```python
from build123d import *

# Parameters (mm, degrees)
BASE_EXTRUDE_DEPTH         = 31.1
SKETCH2_W                  = 13.52
SKETCH2_H                  = 6.37
BOSS_EXTRUDE1_DEPTH        = 8.41
SKETCH3_R                  = 1.545
BASE_MOUNTING_HOLE_1_DEPTH = 35.931591719
SKETCH5_R                  = 1.1305
FACE_MOUNTING_HOLES_DEPTH  = 37.029023023
SHELL_AROUND_PINS_DEPTH    = 5.7
SHELL1_START               = 0.44
SHELL1_DEPTH               = 18.2
SHELL1_START_2             = 8.5
SHELL1_2_OUTLINE_W         = 11.54
SHELL1_2_OUTLINE_H         = 30.22
SHELL1_2_OUTLINE_R         = 1.5705
SHELL1_2_DEPTH             = 4
SHELL1_START_3             = 12.5
SHELL1_3_DEPTH             = 6.14
SHELL1_START_4             = 5.3050001
SHELL1_4_DEPTH             = 3.1949999
SHELL1_5_DEPTH             = 0.8949999
SHELL1_START_5             = 0.09
SHELL1_6_OUTLINE_W         = 5.49
SHELL1_6_OUTLINE_H         = 12.64
SHELL1_6_DEPTH             = 0.35
SHELL1_7_DEPTH             = 2.29
BOSS_EXTRUDE2_DEPTH        = 3.9
BOSS_EXTRUDE3_DEPTH        = 6.24
SKETCH9_R                  = 0.675
CUT_EXTRUDE1_DEPTH         = 6.4


with BuildPart() as part:
    # Sketch1 → Base-Extrude (new body)
    with BuildSketch(Plane.XY):
        Polygon((0, 0), (12.94, 0), (12.94, 12.42), (8.06, 12.42), (8.06, 3.17), (0, 3.17), align=None)
    extrude(amount=BASE_EXTRUDE_DEPTH)

    # Sketch2 → Boss-Extrude1 (add)
    with BuildSketch(Plane.ZY.offset(-8.06)):
        with Locations((15.55, 6.355)):
            Rectangle(SKETCH2_W, SKETCH2_H)
    extrude(amount=BOSS_EXTRUDE1_DEPTH)

    # Sketch3 → Base Mounting Hole 1 (cut, through all)
    with BuildSketch(Plane(origin=(0, 3.17, 0), x_dir=(-1, 0, 0), z_dir=(0, 1, 0))):
        with Locations((-3.32, 3.05)):
            Circle(SKETCH3_R)
        with Locations((-3.32, 28.05)):
            Circle(SKETCH3_R)
    extrude(amount=-BASE_MOUNTING_HOLE_1_DEPTH, mode=Mode.SUBTRACT)

    # Sketch5 → Face Mounting Holes (cut, through all)
    with BuildSketch(Plane(origin=(12.94, 0, 0), x_dir=(0, 0, -1), z_dir=(1, 0, 0))):
        with Locations((-3.05, 6.04)):
            Circle(SKETCH5_R)
        with Locations((-28.05, 6.04)):
            Circle(SKETCH5_R)
    extrude(amount=-FACE_MOUNTING_HOLES_DEPTH, mode=Mode.SUBTRACT)

    # Sketch6 → Shell around Pins (add)
    with BuildSketch(Plane(origin=(12.94, 0, 0), x_dir=(0, 0, -1), z_dir=(1, 0, 0))):
        with BuildLine():
            Line((-22.906967712, 11.06), (-8.213032288, 11.06))
            ThreePointArc((-8.213032288, 11.06), (-7.106786662, 10.573025476), (-6.718825618, 9.428294154))
            Line((-6.718825618, 9.428294154), (-7.309392629, 2.728294154))
            ThreePointArc((-7.309392629, 2.728294154), (-7.790573821, 1.753754374), (-8.803599298, 1.36))
            Line((-8.803599298, 1.36), (-22.316400702, 1.36))
            ThreePointArc((-22.316400702, 1.36), (-23.329426179, 1.753754374), (-23.810607371, 2.728294154))
            Line((-23.810607371, 2.728294154), (-24.401174382, 9.428294154))
            ThreePointArc((-24.401174382, 9.428294154), (-24.013213338, 10.573025476), (-22.906967712, 11.06))
        make_face()
    extrude(amount=SHELL_AROUND_PINS_DEPTH)

    # Shell1: read off the stored shape, not the designer's step
    # Shell1 outline → Shell1 (cut)
    with BuildSketch(Plane.YZ.offset(SHELL1_START)):
        with BuildLine():
            Line((2.73, 21.87), (2.73, 23.368398801))
            ThreePointArc((2.73, 23.368398801), (2.06583377, 23.018469075), (1.8, 22.316400702))
            Line((1.8, 22.316400702), (1.8, 8.803599298))
            ThreePointArc((1.8, 8.803599298), (2.06583377, 8.101530925), (2.73, 7.751601199))
            Line((2.73, 7.751601199), (2.73, 9.23))
            Line((2.73, 9.23), (9.1, 9.23))
            Line((9.1, 9.23), (9.1, 21.87))
            Line((9.1, 21.87), (2.73, 21.87))
        make_face()
    extrude(amount=SHELL1_DEPTH, mode=Mode.SUBTRACT)

    # Shell1 2 outline → Shell1 2 (cut)
    with BuildSketch(Plane.YZ.offset(SHELL1_START_2)):
        with Locations((6.21, 15.55)):
            Rectangle(SHELL1_2_OUTLINE_W, SHELL1_2_OUTLINE_H)
        with Locations((6.04, 3.05)):
            Circle(SHELL1_2_OUTLINE_R, mode=Mode.SUBTRACT)
        with Locations((6.04, 28.05)):
            Circle(SHELL1_2_OUTLINE_R, mode=Mode.SUBTRACT)
        with BuildLine():
            ThreePointArc((1.8, 22.316400702), (2.06583377, 23.018469075), (2.73, 23.368398801))
            Line((2.73, 23.368398801), (2.73, 21.87))
            Line((2.73, 21.87), (9.1, 21.87))
            Line((9.1, 21.87), (9.1, 9.23))
            Line((9.1, 9.23), (2.73, 9.23))
            Line((2.73, 9.23), (2.73, 7.751601199))
            ThreePointArc((2.73, 7.751601199), (2.06583377, 8.101530925), (1.8, 8.803599298))
            Line((1.8, 8.803599298), (1.8, 22.316400702))
        make_face(mode=Mode.SUBTRACT)
    extrude(amount=SHELL1_2_DEPTH, mode=Mode.SUBTRACT)

    # Shell1 3 outline → Shell1 3 (cut)
    with BuildSketch(Plane.YZ.offset(SHELL1_START_3)):
        with BuildLine():
            ThreePointArc((2.766927869, 23.372306748), (2.74844682, 23.370514495), (2.73, 23.368398801))
            Line((2.73, 23.368398801), (2.73, 21.87))
            Line((2.73, 21.87), (9.1, 21.87))
            Line((9.1, 21.87), (9.1, 9.23))
            Line((9.1, 9.23), (2.73, 9.23))
            Line((2.73, 9.23), (2.73, 7.751601199))
            ThreePointArc((2.73, 7.751601199), (2.74844682, 7.749485505), (2.766927869, 7.747693252))
            Line((2.766927869, 7.747693252), (9.466927869, 7.157126241))
            ThreePointArc((9.466927869, 7.157126241), (10.275871337, 7.431285379), (10.62, 8.213032288))
            Line((10.62, 8.213032288), (10.62, 22.906967712))
            ThreePointArc((10.62, 22.906967712), (10.275871337, 23.688714621), (9.466927869, 23.962873759))
            Line((9.466927869, 23.962873759), (2.766927869, 23.372306748))
        make_face()
    extrude(amount=SHELL1_3_DEPTH, mode=Mode.SUBTRACT)

    # Shell1 4 outline → Shell1 4 (cut)
    with BuildSketch(Plane.YZ.offset(SHELL1_START_4)):
        with BuildLine():
            Line((2.73, 23.368398801), (2.73, 30.66))
            Line((2.73, 30.66), (0.44, 30.66))
            Line((0.44, 30.66), (0.44, 0.44))
            Line((0.44, 0.44), (2.73, 0.44))
            Line((2.73, 0.44), (2.73, 7.751601199))
            ThreePointArc((2.73, 7.751601199), (2.06583377, 8.101530925), (1.8, 8.803599298))
            Line((1.8, 8.803599298), (1.8, 22.316400702))
            ThreePointArc((1.8, 22.316400702), (2.06583377, 23.018469075), (2.73, 23.368398801))
        make_face()
    extrude(amount=SHELL1_4_DEPTH, mode=Mode.SUBTRACT)

    # Shell1 5 outline → Shell1 5 (cut)
    with BuildSketch(Plane.YZ.offset(SHELL1_START)):
        with BuildLine():
            Line((2.73, 23.368398801), (2.73, 30.66))
            Line((2.73, 30.66), (0.44, 30.66))
            Line((0.44, 30.66), (0.44, 0.44))
            Line((0.44, 0.44), (2.73, 0.44))
            Line((2.73, 0.44), (2.73, 7.751601199))
            ThreePointArc((2.73, 7.751601199), (2.06583377, 8.101530925), (1.8, 8.803599298))
            Line((1.8, 8.803599298), (1.8, 22.316400702))
            ThreePointArc((1.8, 22.316400702), (2.06583377, 23.018469075), (2.73, 23.368398801))
        make_face()
    extrude(amount=SHELL1_5_DEPTH, mode=Mode.SUBTRACT)

    # Shell1 6 outline → Shell1 6 (cut)
    with BuildSketch(Plane.YZ.offset(SHELL1_START_5)):
        with Locations((6.355, 15.55)):
            Rectangle(SHELL1_6_OUTLINE_W, SHELL1_6_OUTLINE_H)
    extrude(amount=SHELL1_6_DEPTH, mode=Mode.SUBTRACT)

    # Shell1 7 outline → Shell1 7 (cut)
    with BuildSketch(Plane(origin=(0, 0, 0), x_dir=(1, 0, 0), z_dir=(0, 1, 0)).offset(SHELL1_START)):
        with BuildLine():
            Line((1.335, -28.05), (1.3349999, -30.66))
            Line((1.3349999, -30.66), (5.3050001, -30.66))
            Line((5.3050001, -30.66), (5.305, -28.05))
            ThreePointArc((5.305, -28.05), (3.32, -30.035), (1.335, -28.05))
        make_face()
        with BuildLine():
            Line((1.335, -3.049999981), (1.335, -28.05))
            ThreePointArc((1.335, -28.05), (3.32, -26.065), (5.305, -28.05))
            Line((5.305, -28.05), (5.305, -3.05))
            ThreePointArc((5.305, -3.05), (3.31999999, -5.035), (1.335, -3.049999981))
        make_face()
        with BuildLine():
            Line((1.3349999, -0.44), (1.335, -3.049999981))
            ThreePointArc((1.335, -3.049999981), (3.32000001, -1.065), (5.305, -3.05))
            Line((5.305, -3.05), (5.3050001, -0.44))
            Line((5.3050001, -0.44), (1.3349999, -0.44))
        make_face()
    extrude(amount=SHELL1_7_DEPTH, mode=Mode.SUBTRACT)

    # Sketch7 → Boss-Extrude2 (add)
    with BuildSketch(Plane(origin=(8.5, 0, 0), x_dir=(0, 0, -1), z_dir=(1, 0, 0))):
        with BuildLine():
            Line((-22.235829146, 1.8), (-8.884170854, 1.8))
            ThreePointArc((-8.884170854, 1.8), (-8.10887823, 2.10134964), (-7.740618755, 2.84718824))
            Line((-7.740618755, 2.84718824), (-7.165562656, 9.371216493))
            ThreePointArc((-7.165562656, 9.371216493), (-7.462478522, 10.247306751), (-8.309114756, 10.62))
            Line((-8.309114756, 10.62), (-22.810885244, 10.62))
            ThreePointArc((-22.810885244, 10.62), (-23.657521478, 10.247306751), (-23.954437344, 9.371216493))
            Line((-23.954437344, 9.371216493), (-23.379381245, 2.84718824))
            ThreePointArc((-23.379381245, 2.84718824), (-23.01112177, 2.10134964), (-22.235829146, 1.8))
        make_face()
    extrude(amount=BOSS_EXTRUDE2_DEPTH)

    # Sketch8 → Boss-Extrude3 (add)
    with BuildSketch(Plane(origin=(12.4, 0, 0), x_dir=(0, 0, -1), z_dir=(1, 0, 0))):
        with BuildLine():
            Line((-22.235829146, 1.8), (-8.884170854, 1.8))
            ThreePointArc((-8.884170854, 1.8), (-8.10887823, 2.10134964), (-7.740618755, 2.84718824))
            Line((-7.740618755, 2.84718824), (-7.165562656, 9.371216493))
            ThreePointArc((-7.165562656, 9.371216493), (-7.462478522, 10.247306751), (-8.309114756, 10.62))
            Line((-8.309114756, 10.62), (-22.810885244, 10.62))
            ThreePointArc((-22.810885244, 10.62), (-23.657521478, 10.247306751), (-23.954437344, 9.371216493))
            Line((-23.954437344, 9.371216493), (-23.379381245, 2.84718824))
            ThreePointArc((-23.379381245, 2.84718824), (-23.01112177, 2.10134964), (-22.235829146, 1.8))
        make_face()
    extrude(amount=BOSS_EXTRUDE3_DEPTH)

    # Sketch9 → Cut-Extrude1 (cut)
    with BuildSketch(Plane(origin=(18.64, 0, 0), x_dir=(0, 0, -1), z_dir=(1, 0, 0))):
        with Locations((-21.076586145, 7.934935328)):
            Circle(SKETCH9_R)
        with Locations((-18.276586145, 7.934935328)):
            Circle(SKETCH9_R)
        with Locations((-15.476586145, 7.934935328)):
            Circle(SKETCH9_R)
        with Locations((-12.676586145, 7.934935328)):
            Circle(SKETCH9_R)
        with Locations((-9.876586145, 7.934935328)):
            Circle(SKETCH9_R)
        with Locations((-19.731423712, 4.86314649)):
            Circle(SKETCH9_R)
        with Locations((-16.931423712, 4.86314649)):
            Circle(SKETCH9_R)
        with Locations((-14.131423712, 4.86314649)):
            Circle(SKETCH9_R)
        with Locations((-11.331423712, 4.86314649)):
            Circle(SKETCH9_R)
    extrude(amount=-CUT_EXTRUDE1_DEPTH, mode=Mode.SUBTRACT)


solid = part.part
```
Work out the finished part from the listing and answer in its coordinate system (mm). A direction names the side the tool comes from. Round coordinates to 2 decimals unless told otherwise and drop trailing zeros. Order: outer loops, then holes, each group sorted by start corner. A loop starts at its lowest first (then second) coordinate and runs counter-clockwise, first axis right, second up.
Q1. A cutting plane is placed at C-C, the plane x = 6.25. Determine the outline of the cut face in (y, z), then the cut area to 3 significant figures.
Solution:
outline: (0, 0) - (3.17, 0) - (3.17, 8.79) - (9.54, 8.79) - (9.54, 22.31) - (3.17, 22.31) - (3.17, 31.1) - (0, 31.1) - close; hole (0.44, 0.44) - (2.73, 0.44) - (2.73, 9.23) - (9.1, 9.23) - (9.1, 21.87) - (2.73, 21.87) - (2.73, 30.66) - (0.44, 30.66) - close
area: 35.0 mm2
Q2. A tool of negligible diameter and unlimited length cuts with its end or side. For faces 5 (the cylindrical face through (15.48, 4.6, 16.31)), 6 (the flat face through (6, 0.44, 15)), 7 (the cylindrical face through (4.46, 1.61, 29.09)), from which of +Z, -Z, +X, -X, +Y, -Y can it reach the whole face along a straight path? Write none if from no direction.
Solution:
face 5: +X
face 6: none
face 7: +Y, -Y
Q3. Given pin 1 Ø1.9 at (x, y) = (5, 6) entering from +Z; pin 2 Ø3 at (x, y) = (14.5, 8.5) entering from +Z; pin 3 Ø6.5 at (x, z) = (2, 13) entering from +Y, each flat-ended and moving along its own axis, determine where each tip first touches the part or whether it passes through.
Solution:
pin 1: stops at z = 22.31
pin 2: stops at z = 24.41
pin 3: stops at y = 9.54
Q4. A cutting plane is placed at B-B, the plane z = 3.05. Determine the outline of the cut face in (x, y) (1 decimal), then the cut area to 3 significant figures.
Solution:
outline: (0, 0) - (1.8, 0) - (1.8, 3.2) - (0, 3.2) - close; (4.9, 0) - (12.9, 0) - (12.9, 4.9) - (8.1, 4.9) - (8.1, 3.2) - (4.9, 3.2) - close; (8.1, 7.2) - (12.9, 7.2) - (12.9, 12.4) - (8.1, 12.4) - close; hole (0.4, 0.4) - (1.3, 0.4) - (1.3, 2.7) - (0.4, 2.7) - close; hole (5.3, 0.4) - (12.5, 0.4) - (12.5, 4.5) - (8.5, 4.5) - (8.5, 2.7) - (5.3, 2.7) - close; hole (8.5, 7.6) - (12.5, 7.6) - (12.5, 12) - (8.5, 12) - close
area: 22.4 mm2
Q5. The mould has two halves that part along Y. Classify faces 1 (the cylindrical face through (15.485, 4.893, 20.406)), 2 (the flat face through (15.75, 6.13, 7.01)), 3 (the flat face through (10, 1.8, 16)), 4 (the flat face through (8.06, 10, 15)): pulls with the +Y half, pulls with the -Y half, needs draft (parallel to the pull), parting line crosses it, or undercut.
Solution:
face 1: undercut
face 2: pulls with the -Y half
face 3: undercut
face 4: needs draft
Q6. Find the intervals of material crossed by line 1 along Y through (x, z) = (10, 10); line 2 along X through (y, z) = (1, 28); line 3 along Z through (x, y) = (3.32, 2.5) (3 decimals), in increasing order.
Solution:
line 1: y = 0 to 0.44, 1.8 to 10.62, 11.98 to 12.42
line 2: x = 0 to 0.44, 1.34 to 1.78, 4.86 to 5.3, 12.5 to 12.94
line 3: z = 0 to 0.44, 1.065 to 1.505, 4.595 to 5.035, 26.065 to 26.505, 29.595 to 30.035, 30.66 to 31.1
Q7. A cutting plane is placed at A-A, the plane x = 3.32. Count the separate pieces of the cut face and the enclosed holes in it, then the cut area to 3 significant figures.
Solution:
separate pieces: 3
enclosed holes: 3
area: 33.6 mm2
